Answer from the drawing. Dimensions are ordinates in mm from the lowest x, y and z of the part. Give positions to 0.01 mm unless a question says otherwise; leave off trailing zeros. Write each loop counter-clockwise with the first axis right and the second up, starting at its lowest first coordinate (ties: lowest second). Pieces come first, ordered by that corner, then holes. Notation, with made-up numbers: (37, -7) -> (89, -7) arc R10 cw to (89, -1) -> close; hole circle Ø3 at (53, -2.5). An arc over 180 degrees is marked (long way). Write item = value, one per line.
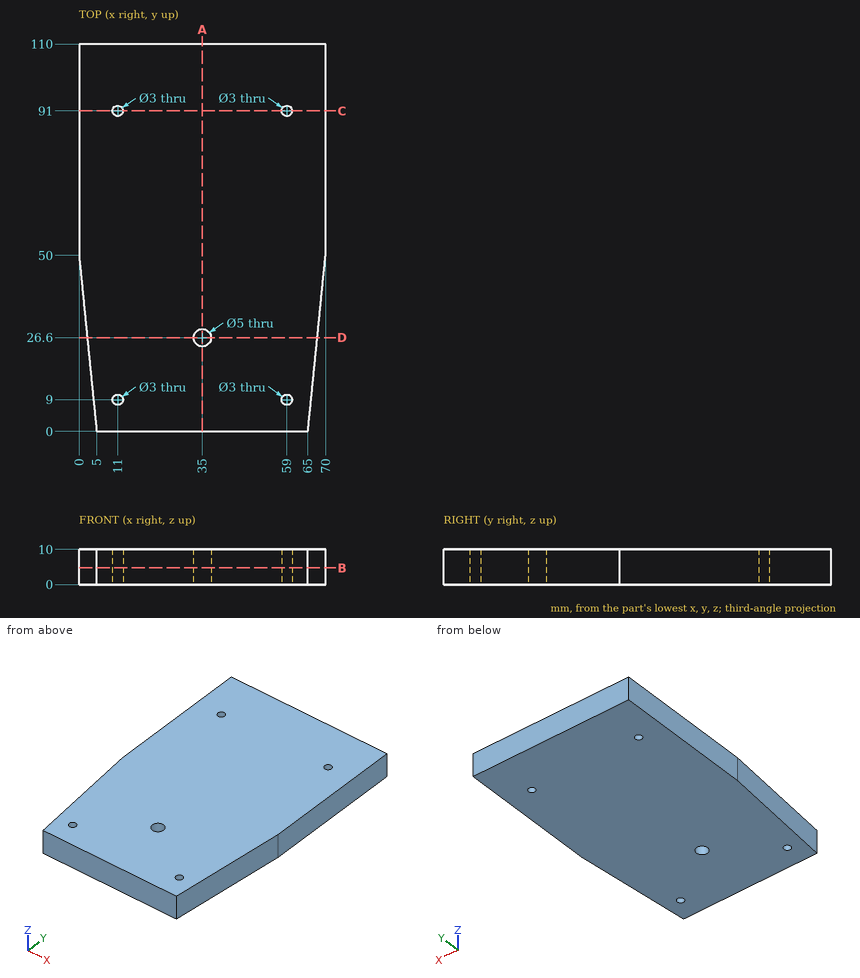
(1) The part is cut by section B-B on z = 4.75. Determine the outline of the cut face in (x, y), plus the area to 3 significant figures.
Checks:
outline = (0, 50) -> (5, 0) -> (65, 0) -> (70, 50) -> (70, 110) -> (0, 110) -> close; hole circle Ø3 at (11, 9); hole circle Ø3 at (11, 91); hole circle Ø5 at (35, 26.6); hole circle Ø3 at (59, 9); hole circle Ø3 at (59, 91)
area = 7,400 mm²
(2) Consider L1, parallel to Y at x = 59, z = 4; L2, parallel to Y at x = 35, z = 4.25; L3, parallel to X at y = 91, z = 6. Determine where each line is inside the solid, lowest interval first.
Checks:
L1 = 0 to 7.5, 10.5 to 89.5, 92.5 to 110
L2 = 0 to 24.1, 29.1 to 110
L3 = 0 to 9.5, 12.5 to 57.5, 60.5 to 70
(3) The part is cut by section D-D on y = 26.6. Determine the outline of the cut face in (x, z), plus the area to 3 significant figures.
Checks:
outline = (2.34, 0) -> (32.5, 0) -> (32.5, 10) -> (2.34, 10) -> close; (37.5, 0) -> (67.66, 0) -> (67.66, 10) -> (37.5, 10) -> close
area = 603 mm²
(4) The part is cut by section C-C on y = 91. Determine the outline of the cut face in (x, z).
Checks:
outline = (0, 0) -> (9.5, 0) -> (9.5, 10) -> (0, 10) -> close; (12.5, 0) -> (57.5, 0) -> (57.5, 10) -> (12.5, 10) -> close; (60.5, 0) -> (70, 0) -> (70, 10) -> (60.5, 10) -> close
(5) Given P1, Ø4, axis at y = 40, z = 3.5, coming from the -X side; P2, Ø4, axis at x = 11, y = 9, coming from the -Z side; P3, Ø2.5, axis at x = 11, y = 91, coming from the +Z side; P4, Ø3, axis at y = 46, z = 2.5, coming from the +X side, each flat-ended and moving along its own axis, determine where each tip first touches the part or whether it passes through.
Checks:
P1 = 0.8
P2 = 0
P3 = through
P4 = 69.75
(6) The part is cut by section A-A on x = 35. Determine the outline of the cut face in (y, z).
Checks:
outline = (0, 0) -> (24.1, 0) -> (24.1, 10) -> (0, 10) -> close; (29.1, 0) -> (110, 0) -> (110, 10) -> (29.1, 10) -> close
